from build123d import *

# Parameters (mm, degrees)
SKETCH_1_R      = 1.45
EXTRUDE_1_DEPTH = 3
FILLET_1_R      = 3


with BuildPart() as part:
    # 草图1 → 凸台-拉伸1 (new body)
    with BuildSketch(Plane(origin=(0, 0, 0), x_dir=(1, 0, 0), z_dir=(0, 1, 0))):
        Polygon((-200, 25), (-185, 25), (-169.545454545, 23.052363238), (-160.024381788, 11.461454148), (-175.478927243, -1.233309529), (-185, -9.054165144), (-200, -9.054165144), (-200, -4.917341068), align=None)
        with Locations(Location((-176.375827258, 7.735835936, 0), (0, 0, 270))):
            Circle(SKETCH_1_R, mode=Mode.SUBTRACT)
        with Locations(Location((-168.648554531, 14.083217774, 0), (0, 0, 270))):
            Circle(SKETCH_1_R, mode=Mode.SUBTRACT)
        with Locations(Location((-192.5, 20, 0), (0, 0, 270))):
            Circle(SKETCH_1_R, mode=Mode.SUBTRACT)
        with Locations(Location((-192.5, 10, 0), (0, 0, 270))):
            Circle(SKETCH_1_R, mode=Mode.SUBTRACT)
    extrude(amount=EXTRUDE_1_DEPTH)

    # 圆角1
    fillet_1_edges = [part.edges().sort_by_distance(p)[0] for p in [
        (-185, 1.5, 9.054165144),
        (-200, 1.5, 9.054165144),
        (-200, 1.5, -25),
        (-185, 1.5, -25),
        (-169.545454545, 1.5, -23.052363238),
        (-160.024381788, 1.5, -11.461454148),
    ]]
    fillet(fillet_1_edges, radius=FILLET_1_R)


solid = part.part
The listing builds one solid part. Answer for the finished solid, in the listing's coordinates (mm). Give positions to 0.01 mm unless a question says otherwise; leave off trailing zeros. Loops run counter-clockwise (first coordinate to the right, second up) from the corner with the lowest first, then second, coordinate; pieces in that order, holes last.
Item 1: Determine the mould class of faces 1 (the flat face through (-185, 0, -8)), 2 (the cylindrical face through (-174.938, 1.479, -7.925)), 3 (the cylindrical face through (-199.145, 1.521, 8.152)), 4 (the flat face through (-165.406, 1.479, -18.013)) for opening direction X: +X half, -X half, draft (parallel to the pull), parting line (faces both ways), or undercut.
Derived:
face 1: draft
face 2: undercut
face 3: -X half
face 4: +X half
Item 2: A cutting plane is placed at C-C (y = 2.25). Give the vertices of the cut face in (x, z).
Derived:
outline: (-200, -22) arc R3 ccw to (-197, -25) - (-185.19, -25) arc R3 ccw to (-184.81, -24.98) - (-170.73, -23.2) arc R3 ccw to (-168.79, -22.13) - (-161.93, -13.78) arc R3 ccw to (-162.34, -9.56) - (-184.17, 8.37) arc R3 ccw to (-186.07, 9.05) - (-197, 9.05) arc R3 ccw to (-200, 6.05) - close; hole circle Ø2.9 at (-192.5, -20); hole circle Ø2.9 at (-192.5, -10); hole circle Ø2.9 at (-176.38, -7.74); hole circle Ø2.9 at (-168.65, -14.08)
Item 3: This flat-tipped pin is pushed along its axis until it touches: pin 1 Ø4.5 at (x, z) = (-192.5, -20) entering from +Y. Where does it stop, or does it pass through?
Derived:
pin 1: stops at y = 3
Item 4: A cutting plane is placed at A-A (x = -192.5). Give the vertices of the cut face in (y, z).
Derived:
outline: (0, -25) - (3, -25) - (3, -21.45) - (0, -21.45) - close; (0, -18.55) - (3, -18.55) - (3, -11.45) - (0, -11.45) - close; (0, -8.55) - (3, -8.55) - (3, 9.05) - (0, 9.05) - close
Item 5: Find the intervals of material crossed by line 1 along Z through (x, y) = (-192.5, 1.7); line 2 along X through (y, z) = (0.65, -9); line 3 along X through (y, z) = (2.45, -10), in increasing order.
Derived:
line 1: z = -25 to -21.45, -18.55 to -11.45, -8.55 to 9.05
line 2: x = -200 to -193.55, -191.45 to -177.09, -175.67 to -163.02
line 3: x = -200 to -193.95, -191.05 to -161.91
Item 6: A cutting plane is placed at B-B (z = -10.5). Give the vertices of the cut face in (x, y).
Derived:
outline: (-200, 0) - (-193.86, 0) - (-193.86, 3) - (-200, 3) - close; (-191.14, 0) - (-161.58, 0) - (-161.58, 3) - (-191.14, 3) - close
Item 7: A cutting plane is placed at D-D (z = -15). Give the vertices of the cut face in (x, y).
Derived:
outline: (-200, 0) - (-169.77, 0) - (-169.77, 3) - (-200, 3) - close; (-167.53, 0) - (-162.93, 0) - (-162.93, 3) - (-167.53, 3) - close
